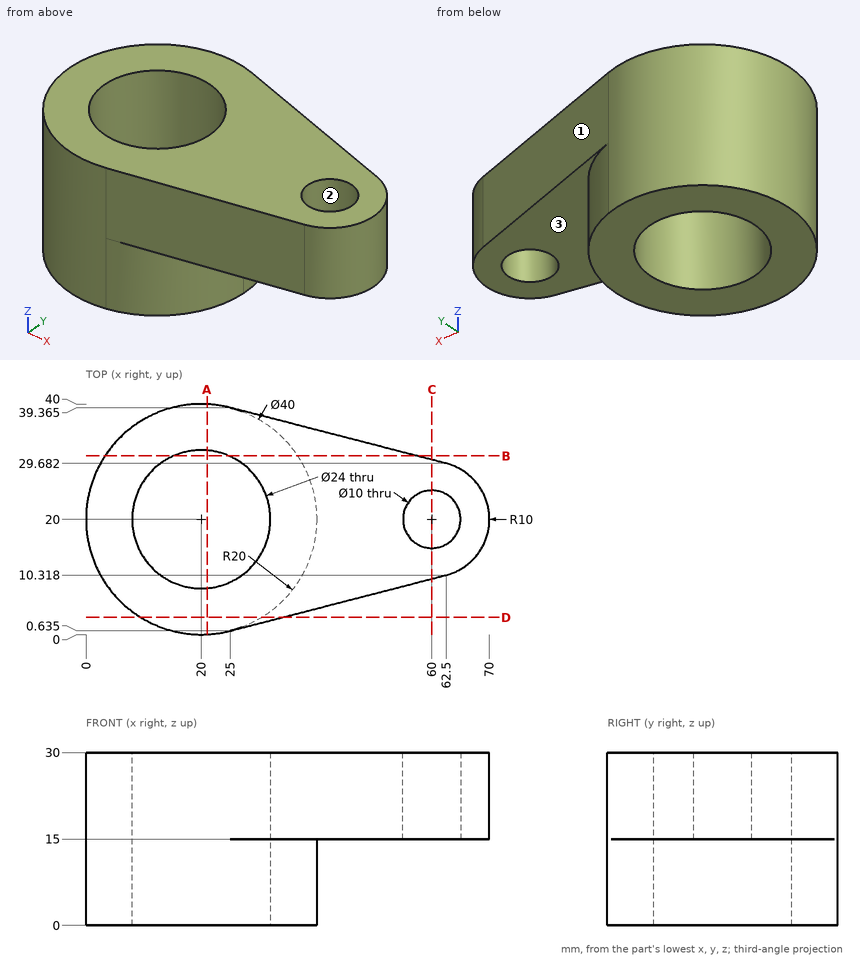
Answer from the drawing. Dimensions are ordinates in mm from the lowest x, y and z of the part. Coordinates: 2 decimals unless noted, no trailing zeros. Order: outer loops, then holes, each group sorted by start corner. A loop starts at its lowest first (then second) coordinate and runs counter-clockwise, first axis right, second up. Notation, with made-up numbers: (-5.5, 30) - (0.5, 30) arc R33 cw to (0.5, 62) - close; hole circle Ø7 at (-36, -20). An arc over 180 degrees is marked (long way). Put each result on its own line as item: value. Start each with the question number.
1) Find section D-D (y = 3). Give the vertices of the cut face in (x, z) (1 decimal).
2) For a pull along Y with two mould halves and no side action, classify the marked faces 1, 2 and 3 as released by +Y, released by -Y, zero draft, split by the parting line, or undercut.
3) Find section A-A (x = 21). Give the vertices of the cut face in (y, z) (1 decimal), plus the area to 3 significant figures.
4) Flat-ended cylindrical pins translate along their axes: pin 1 (3 mm diameter, centred on y = 7.5, z = 3, fed in from +X); pin 2 (3 mm diameter, centred on y = 7, z = 13, fed in from +X); pin 3 (10 mm diameter, centred on x = 46.5, y = 16.5, fed in from -Z). Find the tip coordinate at first contact, or state that the pin passes through.
5) Find section C-C (x = 60). Give the vertices of the cut face in (y, z).
6) Find the intervals of material crossed by line 1 (Y direction, x = 20, z = 18); line 2 (X direction, y = 16, z = 28) (1 decimal); line 3 (X direction, y = 23.5, z = 24.25) (1 decimal), in increasing order. Write a range as from..to.
7) Find section B-B (y = 31). Give the vertices of the cut face in (x, z) (1 decimal), plus the area to 4 significant figures.
Results list:
1. outline: (9.5, 0) - (30.5, 0) - (30.5, 15) - (34.2, 15) - (34.2, 30) - (9.5, 30) - close
2. face 1: released by +Y
2. face 2: undercut
2. face 3: zero draft
3. outline: (0, 0) - (8, 0) - (8, 30) - (0, 30) - close; (32, 0) - (40, 0) - (40, 30) - (32, 30) - close
3. area: 481 mm^2
4. pin 1: stops at x = 36.7
4. pin 2: stops at x = 36.36
4. pin 3: stops at z = 15
5. outline: (9.67, 15) - (15, 15) - (15, 30) - (9.67, 30) - close; (25, 15) - (30.33, 15) - (30.33, 30) - (25, 30) - close
6. line 1: y = 0..8, 32..40
6. line 2: x = 0.4..8.7, 31.3..57, 63..69.2
6. line 3: x = 0.3..8.5, 31.5..56.4, 63.6..69.4
7. outline: (3.3, 0) - (15.2, 0) - (15.2, 30) - (3.3, 30) - close; (24.8, 0) - (36.7, 0) - (36.7, 15) - (57.4, 15) - (57.4, 30) - (24.8, 30) - close
7. area: 1,025 mm^2
